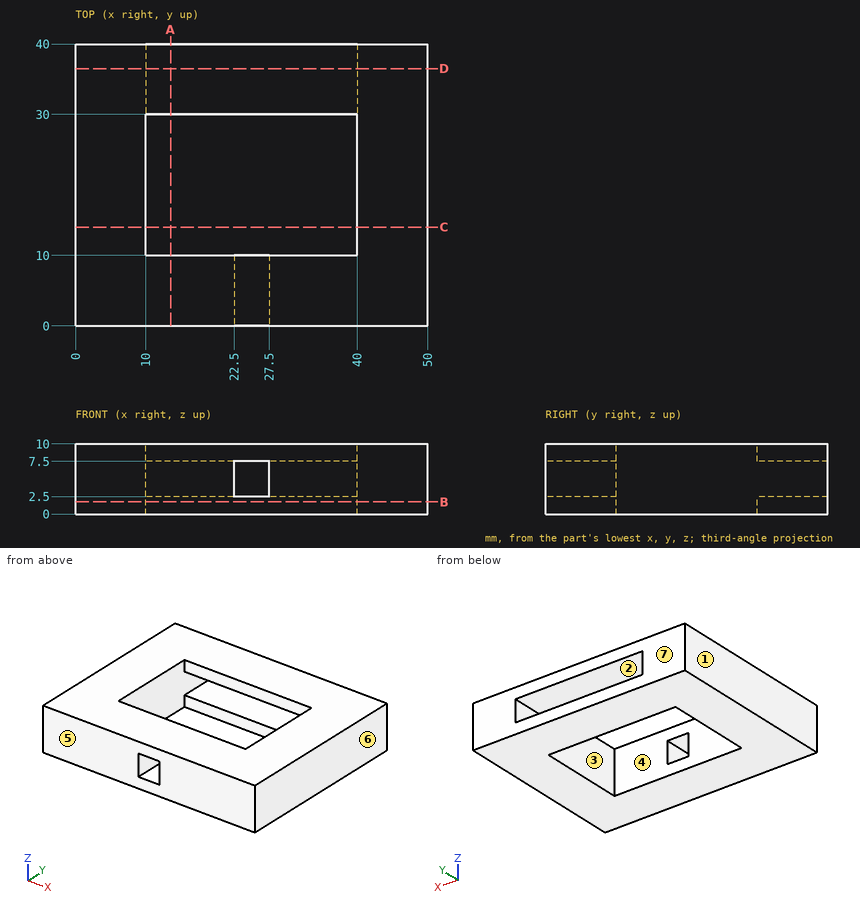
Geometry check sheet. Reference: drawing and pictorial views, mm from the part's lowest x, y, z. A direction names the side the tool comes from. Give positions to 0.01 mm unless a question says otherwise; leave off trailing zeros. Loops run counter-clockwise (first coordinate to the right, second up) from the corner with the lowest first, then second, coordinate; pieces in that order, holes last. Notation, with made-up numbers: (-9, 15) - (46, 15) arc R21 ccw to (46, 42) - close; hole circle Ø11 at (42, -37.75). An arc over 180 degrees is marked (long way). Use CSV: the item, a comma, the result in double quotes. Start each with the question number.
Q1. Section check B-B, the plane z = 1.75. Record the cut outline in (x, y), and give its area (3 significant figures).
Q2. Access from +Z, -Z, +X, -X, +Y, -Y to the whole of each face (thin tool, end or side, straight path). Record for the marked faces 1, 2 and 3.
Q3. Section check A-A, the plane x = 13.5. Record the cut outline in (y, z), and give its area (3 significant figures).
Q4. Scan lines: probe 1 along X at (y, z) = (13, 7); probe 2 along Y at (x, z) = (35, 8); probe 3 along Y at (x, z) = (35.5, 3.5). Record each from-to range of solid material in increasing order. Write a range as from..to.
Q5. Section check D-D, the plane y = 36.5. Record the cut outline in (x, z).
Q6. Section check C-C, the plane y = 14. Record the cut outline in (x, z), and give its area (3 significant figures).
Q7. Release check for a two-part mould opening along Y. For the marked faces 4, 5, 6 and 7 record: +Y half, -Y half, draft (parallel to the pull), parting line (faces both ways), or undercut.
Findings below:
1,outline,"(0, 0) - (50, 0) - (50, 40) - (0, 40) - close; hole (10, 10) - (40, 10) - (40, 30) - (10, 30) - close"
1,area,"1,400 mm^2"
2,face 1,"+Z, -Z, -X, +Y, -Y"
2,face 2,"+Y"
2,face 3,"none"
3,outline,"(0, 0) - (10, 0) - (10, 10) - (0, 10) - close; (30, 0) - (40, 0) - (40, 2.5) - (30, 2.5) - close; (30, 7.5) - (40, 7.5) - (40, 10) - (30, 10) - close"
3,area,"150 mm^2"
4,probe 1,"x = 0..10, 40..50"
4,probe 2,"y = 0..10, 30..40"
4,probe 3,"y = 0..10"
5,outline,"(0, 0) - (50, 0) - (50, 10) - (0, 10) - close; hole (10, 2.5) - (40, 2.5) - (40, 7.5) - (10, 7.5) - close"
6,outline,"(0, 0) - (10, 0) - (10, 10) - (0, 10) - close; (40, 0) - (50, 0) - (50, 10) - (40, 10) - close"
6,area,"200 mm^2"
7,face 4,"undercut"
7,face 5,"-Y half"
7,face 6,"draft"
7,face 7,"+Y half"
